Part model, mm, in its own coordinate system. Coordinates: 2 decimals unless noted, no trailing zeros. Write each loop counter-clockwise with the first axis right and the second up, starting at its lowest first coordinate (ties: lowest second). Pieces come first, ordered by that corner, then holes. Notation, with made-up numbers: (52, -33.5) - (88, -33.5) arc R19 ccw to (88, -6.5) - close; hole circle Ø6 at (-36, -6). An arc over 180 degrees is marked (long way). Use a Markdown table: item, result.
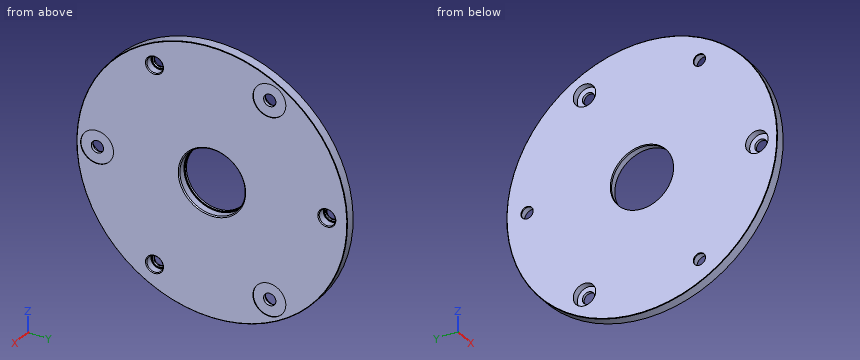
```python
from build123d import *

# Parameters (mm, degrees)
SKETCH2_R                       = 66.25
SKETCH2_R_2                     = 16
BOSS_EXTRUDE1_DEPTH             = 5
SKETCH4_R                       = 3
CUT_EXTRUDE1_DEPTH              = 5
SKETCH4_3_R                     = 4
SKETCH4_3_R_2                   = 3
CUT_EXTRUDE2_DEPTH              = 4
CHAMFER1_SIZE                   = 0.4
FILLET3_R                       = 0.2
SKETCH5_R                       = 8.05
CUT_EXTRUDE3_DEPTH              = 0.3
CBORE_FOR_M6_SBHCS1_D           = 6
CBORE_FOR_M6_SBHCS1_CBORE_D     = 11
CBORE_FOR_M6_SBHCS1_CBORE_DEPTH = 3.3
CIRPATTERN1_COUNT               = 3
CHAMFER1_OF_CIRPATTERN1_SIZE    = 0.4
FILLET3_OF_CIRPATTERN1_R        = 0.2
BOSS_EXTRUDE2_START             = -5
SKETCH8_R                       = 16
SKETCH8_R_2                     = 15.5
BOSS_EXTRUDE2_DEPTH             = 1
FILLET2_R                       = 0.2
CHAMFER2_SIZE                   = 0.5
CHAMFER3_SIZE                   = 0.2


with BuildPart() as part:
    # Sketch2 → Boss-Extrude1 (new body)
    with BuildSketch(Plane(origin=(0, 0, 0), x_dir=(0, 0, -1), z_dir=(1, 0, 0))):
        Circle(SKETCH2_R)
        Circle(SKETCH2_R_2, mode=Mode.SUBTRACT)
    extrude(amount=-BOSS_EXTRUDE1_DEPTH)

    # Sketch4 → Cut-Extrude1 (cut)
    with BuildSketch(Plane(origin=(0, 0, 0), x_dir=(0, 0, -1), z_dir=(1, 0, 0))):
        with Locations((0, 56.25)):
            Circle(SKETCH4_R)
    cut_extrude1 = extrude(amount=-CUT_EXTRUDE1_DEPTH, mode=Mode.SUBTRACT)

    # Sketch4<3> → Cut-Extrude2 (cut)
    with BuildSketch(Plane(origin=(0, 0, 0), x_dir=(0, 0, -1), z_dir=(1, 0, 0))):
        with Locations((0, 56.25)):
            Circle(SKETCH4_3_R)
        with Locations((0, 56.25)):
            Circle(SKETCH4_3_R_2, mode=Mode.SUBTRACT)
    cut_extrude2 = extrude(amount=-CUT_EXTRUDE2_DEPTH, mode=Mode.SUBTRACT)

    # Chamfer1
    chamfer1_edges = [part.edges().sort_by_distance(p)[0] for p in [
        (0, 56.25, 4),
        (-4, 56.25, 3),
    ]]
    chamfer(chamfer1_edges, length=CHAMFER1_SIZE)

    # Fillet3
    fillet3_edges = [part.edges().sort_by_distance(p)[0] for p in [
        (-4, 56.25, 4),
    ]]
    fillet(fillet3_edges, radius=FILLET3_R)

    # Sketch5 → Cut-Extrude3 (cut)
    with BuildSketch(Plane(origin=(0, 0, 0), x_dir=(0, 0, -1), z_dir=(1, 0, 0))):
        with Locations((48.713928963, 28.125)):
            Circle(SKETCH5_R)
    cut_extrude3 = extrude(amount=-CUT_EXTRUDE3_DEPTH, mode=Mode.SUBTRACT)

    # CBORE for M6 SBHCS1 (through all)
    with Locations(Plane.ZY.offset(5)):
        with Locations((-48.713928963, 28.125)):
            cbore_for_m6_sbhcs1 = CounterBoreHole(CBORE_FOR_M6_SBHCS1_D / 2, CBORE_FOR_M6_SBHCS1_CBORE_D / 2, CBORE_FOR_M6_SBHCS1_CBORE_DEPTH)

    # CirPattern1: Cut-Extrude1, Cut-Extrude2, Cut-Extrude3, CBORE for M6 SBHCS1 ×3 about axis
    cirpattern1_axis = Axis((0, 0, 0), (1, 0, 0))
    for i in range(1, CIRPATTERN1_COUNT):
        add(cut_extrude1.rotate(cirpattern1_axis, i * 360 / CIRPATTERN1_COUNT), mode=Mode.SUBTRACT)
        add(cut_extrude2.rotate(cirpattern1_axis, i * 360 / CIRPATTERN1_COUNT), mode=Mode.SUBTRACT)
        add(cut_extrude3.rotate(cirpattern1_axis, i * 360 / CIRPATTERN1_COUNT), mode=Mode.SUBTRACT)
        add(cbore_for_m6_sbhcs1.rotate(cirpattern1_axis, i * 360 / CIRPATTERN1_COUNT), mode=Mode.SUBTRACT)

    # Chamfer1 of CirPattern1
    chamfer1_of_cirpattern1_edges = [part.edges().sort_by_distance(p)[0] for p in [
        (0, -31.589101615, 46.713928963),
        (-4, -30.723076211, 47.213928963),
        (0, -24.660898385, -50.713928963),
        (-4, -25.526923789, -50.213928963),
    ]]
    chamfer(chamfer1_of_cirpattern1_edges, length=CHAMFER1_OF_CIRPATTERN1_SIZE)

    # Fillet3 of CirPattern1
    fillet3_of_cirpattern1_edges = [part.edges().sort_by_distance(p)[0] for p in [
        (-4, -31.589101615, 46.713928963),
        (-4, -24.660898385, -50.713928963),
    ]]
    fillet(fillet3_of_cirpattern1_edges, radius=FILLET3_OF_CIRPATTERN1_R)

    # Sketch8 → Boss-Extrude2 (add)
    with BuildSketch(Plane(origin=(0, 0, 0), x_dir=(0, 0, -1), z_dir=(1, 0, 0)).offset(BOSS_EXTRUDE2_START)):
        Circle(SKETCH8_R)
        Circle(SKETCH8_R_2, mode=Mode.SUBTRACT)
    extrude(amount=BOSS_EXTRUDE2_DEPTH)

    # Fillet2
    fillet2_edges = [part.edges().sort_by_distance(p)[0] for p in [
        (-4, 0, 16),
    ]]
    fillet(fillet2_edges, radius=FILLET2_R)

    # Chamfer2
    chamfer2_edges = [part.edges().sort_by_distance(p)[0] for p in [
        (0, 0, 16),
    ]]
    chamfer(chamfer2_edges, length=CHAMFER2_SIZE)

    # Chamfer3
    chamfer3_edges = [part.edges().sort_by_distance(p)[0] for p in [
        (0, 0, 66.25),
        (-5, 0, 66.25),
    ]]
    chamfer(chamfer3_edges, length=CHAMFER3_SIZE)


solid = part.part
```
Item 1: Band-saw the part on A-A, the plane y = 0. Give the cut face in (x, z), then the cut area to 3 significant figures.
From the geometry:
| item | result |
|---|---|
| outline | (-5, -66.05) - (-4.8, -66.25) - (-0.2, -66.25) - (0, -66.05) - (0, -16.5) - (-0.5, -16) - (-3.8, -16) arc R0.2 cw to (-4, -15.8) - (-4, -15.5) - (-5, -15.5) - close; (-5, 15.5) - (-4, 15.5) - (-4, 15.8) arc R0.2 cw to (-3.8, 16) - (-0.5, 16) - (0, 16.5) - (0, 66.05) - (-0.2, 66.25) - (-4.8, 66.25) - (-5, 66.05) - close |
| area | 503 mm^2 |
Item 2: Band-saw the part on B-B, the plane z = 0. Count the separate pieces of the cut face and the enclosed holes in it, then the cut area to 3 significant figures.
From the geometry:
| item | result |
|---|---|
| separate pieces | 4 |
| enclosed holes | 0 |
| area | 415 mm^2 |
Item 3: Drop flat-ended pins along their axis: P1, Ø1.5, axis at x = -3, z = -7, coming from the -Y side; P2, Ø7, axis at y = -28.12, z = 48.71, coming from the +X side; P3, Ø8.5, axis at y = -26.5, z = 50.5, coming from the +X side; P4, Ø3.5, axis at y = 26, z = -50, coming from the -X side. Give the stop position or say it passes through.
From the geometry:
| item | result |
|---|---|
| P1 | y = -65.95 |
| P2 | x = -4 |
| P3 | x = 0 |
| P4 | x = -1.7 |
Item 4: Drill centre lines: probe 1 along Y at (x, z) = (-4.75, 0); probe 2 along Z at (x, y) = (-4.4, 1); probe 3 along Y at (x, z) = (-1.25, 0). Where is each one in solid material? Low to high.
From the geometry:
| item | result |
|---|---|
| probe 1 | -66.25 to -61.75, -50.75 to -15.5, 15.5 to 53.25, 59.25 to 66.25 |
| probe 2 | -66.24 to -15.47, 15.47 to 66.24 |
| probe 3 | -66.25 to -59.25, -53.25 to -16, 16 to 52.25, 60.25 to 66.25 |
